Autodesk Inventor part; units mm, degrees
ref_plane "YZ Plane" through (0, 0, 0) normal (1, 0, 0) x (0, 1, 0)
ref_plane "XZ Plane" through (0, 0, 0) normal (0, 1, 0) x (-1, 0, 0)
ref_plane "XY Plane" through (0, 0, 0) normal (0, 0, 1) x (1, 0, 0)
sketch "Sketch1" plane through (0, 0, 0) normal (1, 0, 0) x (0, 1, 0)
  line L0 (128.3979, 81.9005) -> (-112.6021, 81.9005)
  line L1 (-112.6021, 81.9005) -> (-112.6021, -0.0995)
  line L2 (-112.6021, -0.0995) -> (128.3979, -0.0995)
  line L3 (128.3979, -0.0995) -> (128.3979, 81.9005)
  circle A0 centre (-45.6021, 40.9005) radius 19
  line L4 (-112.6021, 73.9005) -> (-109.6021, 73.9005)
  line L5 (-109.6021, 73.9005) -> (-109.6021, 7.9005)
  line L6 (-109.6021, 7.9005) -> (-112.6021, 7.9005)
  line L7 (-112.6021, 7.9005) -> (-112.6021, 73.9005)
  point P0 (0, 0)
  dimension "d0" = 241
  dimension "d1" = 82
  dimension "d2" = 38
  dimension "d3" = 41
  dimension "d4" = 174
  dimension "d5" = 66
  dimension "d6" = 3
  dimension "d7" = 8
extrude "Base" add sketch "Sketch1" along normal blind 5 contours L3 L2 L1 L6 L5 L4 L0
sketch "Sketch2" plane through (5, 0, 0) normal (1, 0, 0) x (0, 0, -1)
  circle A0 centre (-40.9005, -45.6021) radius 19
  circle A1 centre (-65.9005, 108.8979) radius 2.5
  line L0 (-81.9005, 128.3979) -> (-81.9005, -112.6021) construction
  line L1 (0.0995, 128.3979) -> (-81.9005, 128.3979) construction
  line L2 (-81.9005, 128.3979) -> (0.0995, 128.3979) construction
  line L3 (-81.9005, 128.3979) -> (-81.9005, -112.6021) construction
  circle A2 centre (-15.9005, 108.8979) radius 2.5
  circle A3 centre (-65.9005, 58.8979) radius 2.5
  circle A4 centre (-15.9005, 58.8979) radius 2.5
  line L4 (-65.9005, 58.8979) -> (-15.9005, 58.8979) construction
  line L5 (-15.9005, 58.8979) -> (-15.9005, 108.8979) construction
  point P0 (0, 0)
  point P1 (-40.9005, 58.8979)
  dimension "d10" = 5
  dimension "d13" = 50
  dimension "d16" = 50
  dimension "d19" = 19.5
extrude "Bracket holes" cut sketch "Sketch2" against normal up to surface (5 mm away) contours A1 | A2 | A3 | A4
equation "\"d3\" = 0.5 * d1"
equation "\"d7\" = -0.5 * d5 + 0.5 * d1"
properties part number "center wall"
Input: part model. Units: mm. Frame: model coordinates. A direction names the side the tool comes from. Give positions to 0.01 mm unless a question says otherwise; leave off trailing zeros. Order: outer loops, then holes, each group sorted by start corner. A loop starts at its lowest first (then second) coordinate and runs counter-clockwise, first axis right, second up. Notation, with made-up numbers: (-15.75, 62.25) - (34.25, 62.25) arc R23 ccw to (34.25, 93.25) - close; hole circle Ø4 at (47.25, 87.5). An arc over 180 degrees is marked (long way). Put each result on its own line as item: value.
Item 1: Access query for faces 1 (the flat face through (2, -112.602, 4)), 2 (the flat face through (2, -109.602, 41)). Directions: +Z, -Z, +X, -X, +Y, -Y. A direction counts if a zero-diameter tool reaches every point of the face in a straight line with its end or side. Return the directions, or none.
Found:
face 1: +Z, -Z, +X, -X, -Y
face 2: +X, -X, -Y
Item 2: Contact query for a flat-ended pin moving along its axis: pin 1 (2 mm diameter, centred on x = 4.5, z = 48.5, fed in from -Y). Output: stop coordinate, or through.
Found:
pin 1: stops at y = -109.6
Item 3: Draft query along Z for faces 3 (the flat face through (5, 6, 41)), 4 (the flat face through (2, 10, 81.9)), 5 (the cylindrical face through (2.535, 56.457, 16.442)), 6 (the flat face through (2, 6, -0.1)). Return one class per face: +Z half, -Z half, draft (parallel to the pull), parting line (faces both ways), or undercut.
Found:
face 3: draft
face 4: +Z half
face 5: undercut
face 6: -Z half
Item 4: Section query C-C, the plane z = 51. Return loops of the section in (x, y).
Found:
outline: (0, -109.6) - (5, -109.6) - (5, -61.7) - (0, -61.7) - close; (0, -29.51) - (5, -29.51) - (5, 128.4) - (0, 128.4) - close
Item 5: Ray query, L1, parallel to Y at x = 2.65, z = 65.5; L2, parallel to Y at x = 1.5, z = 42; L3, parallel to Y at x = 3.7, z = 70.5. Return the intervals inside material, ascending. Write a range as from..to.
Found:
L1: y = -109.6..56.43, 61.37..106.43, 111.37..128.4
L2: y = -109.6..-64.57, -26.63..128.4
L3: y = -109.6..128.4
Item 6: Section query A-A, the plane z = 37. Return loops of the section in (x, y), then the cut area to 3 significant figures.
Found:
outline: (0, -109.6) - (5, -109.6) - (5, -64.2) - (0, -64.2) - close; (0, -27.01) - (5, -27.01) - (5, 128.4) - (0, 128.4) - close
area: 1,000 mm^2
Item 7: Section query B-B, the plane x = 2.45. Return loops of the section in (y, z), then the cut area to 3 significant figures.
Found:
outline: (-112.6, -0.1) - (128.4, -0.1) - (128.4, 81.9) - (-112.6, 81.9) - (-112.6, 73.9) - (-109.6, 73.9) - (-109.6, 7.9) - (-112.6, 7.9) - close; hole circle Ø38 at (-45.6, 40.9); hole circle Ø5 at (58.9, 15.9); hole circle Ø5 at (58.9, 65.9); hole circle Ø5 at (108.9, 15.9); hole circle Ø5 at (108.9, 65.9)
area: 18,400 mm^2
